CAD build for the part. Positions are in the model's coordinates, mm. Give positions to 0.01 mm unless a question says otherwise; leave off trailing zeros. Loops run counter-clockwise (first coordinate to the right, second up) from the corner with the lowest first, then second, coordinate; pieces in that order, holes last. Notation, with made-up numbers: M 88.5,-38.5 L 128.5,-38.5 A25 ccw 128.5,-18.5 Z; hole C -8.5,-9 d7. An arc over 180 degrees is marked long. Answer as CSV lines item,"result".
from build123d import *

# Parameters (mm, degrees)
F0_W         = 59.3232400715
F0_H         = 118.4509694576
F1_DEPTH     = 7.62
F2_T1_DEPTH  = 33.02
F3_T1_DEPTH  = 33.02
F4_T1_DEPTH  = 33.02
F5_T1_DEPTH  = 33.02
F17_W        = 8.8130328804
F17_H        = 2.5180093944
F18_DEPTH    = 0.254
F19_T1_DEPTH = 1.524
F20_R        = 0.508
F10_R        = 2.8607169915
F21_DEPTH    = 0.254
F11_R        = 2.8607134233
F22_DEPTH    = 0.254
F12_W        = 1.611137297
F12_H        = 7.3773153126
F23_DEPTH    = 0.254
F7_R         = 1.0781434008
F24_DEPTH    = 0.254
F9_W         = 6.8501718342
F9_H         = 1.6440376639
F25_DEPTH    = 0.254
F13_R        = 3.228368755
F26_DEPTH    = 0.254
F14_W        = 1.9021295011
F14_H        = 6.1539448798
F27_DEPTH    = 0.254
F8_R         = 3.0136808832
F28_DEPTH    = 0.254
F6_W         = 58.911472559
F6_H         = 101.9305512309
F29_DEPTH    = 0.254
F16_W        = 8.6615839973
F16_H        = 2.4723988026
F30_DEPTH    = 0.762
F15_R        = 2.8680658163
F31_DEPTH    = 0.762


# Not quite as in the source:
# - a fillet or chamfer that OpenCascade refuses, or shapes differently, is made with other operations: its cross-section is extruded or revolved along the edge and cut away or added


with BuildPart() as f1:
    # F0 (on Front) → F1 (new body)
    with BuildSketch(Plane.XZ):
        Rectangle(F0_W, F0_H)
    extrude(amount=F1_DEPTH)

    # F2: fillet of radius 5.08 on 1 edges, made by hand

    # F2_s2 → F2_t1 (cut)
    with BuildSketch(Plane.XZ.offset(-12.7)):
        with BuildLine():
            add(Edge.make_bspline(
                [(29.6616200358, 54.1454847288), (29.6616200358, 59.2254847288), (24.5816200358, 59.2254847288)],
                knots=[0, 0, 0, 1, 1, 1], degree=2, weights=[1, 1, 1]))
            Line((24.5816200358, 59.2254847288), (29.6616200358, 59.2254847288))
            Line((29.6616200358, 59.2254847288), (29.6616200358, 54.1454847288))
        make_face()
    extrude(amount=F2_T1_DEPTH, mode=Mode.SUBTRACT)

    # F3: fillet of radius 5.08 on 1 edges, made by hand

    # F3_s2 → F3_t1 (cut)
    with BuildSketch(Plane.XZ.offset(-12.7)):
        with BuildLine():
            add(Edge.make_bspline(
                [(-29.6616200358, 54.1454847288), (-29.6616200358, 59.2254847288), (-24.5816200358, 59.2254847288)],
                knots=[0, 0, 0, 1, 1, 1], degree=2, weights=[1, 1, 1]))
            Line((-24.5816200358, 59.2254847288), (-29.6616200358, 59.2254847288))
            Line((-29.6616200358, 59.2254847288), (-29.6616200358, 54.1454847288))
        make_face()
    extrude(amount=F3_T1_DEPTH, mode=Mode.SUBTRACT)

    # F4: fillet of radius 5.08 on 1 edges, made by hand

    # F4_s2 → F4_t1 (cut)
    with BuildSketch(Plane.XZ.offset(-12.7)):
        with BuildLine():
            add(Edge.make_bspline(
                [(-24.5816200358, -59.2254847288), (-29.6616200358, -59.2254847288), (-29.6616200358, -54.1454847288)],
                knots=[0, 0, 0, 1, 1, 1], degree=2, weights=[1, 1, 1]))
            Line((-29.6616200358, -54.1454847288), (-29.6616200358, -59.2254847288))
            Line((-29.6616200358, -59.2254847288), (-24.5816200358, -59.2254847288))
        make_face()
    extrude(amount=F4_T1_DEPTH, mode=Mode.SUBTRACT)

    # F5: fillet of radius 5.08 on 1 edges, made by hand

    # F5_s2 → F5_t1 (cut)
    with BuildSketch(Plane.XZ.offset(-12.7)):
        with BuildLine():
            add(Edge.make_bspline(
                [(29.6616200358, -54.1454847288), (29.6616200358, -59.2254847288), (24.5816200358, -59.2254847288)],
                knots=[0, 0, 0, 1, 1, 1], degree=2, weights=[1, 1, 1]))
            Line((24.5816200358, -59.2254847288), (29.6616200358, -59.2254847288))
            Line((29.6616200358, -59.2254847288), (29.6616200358, -54.1454847288))
        make_face()
    extrude(amount=F5_T1_DEPTH, mode=Mode.SUBTRACT)

    # F17 (on face) → F18 (join)
    with BuildSketch(Plane.XY.offset(59.2254847288)):
        with Locations((18.3535870165, -3.5715140402)):
            Rectangle(F17_W, F17_H)
    extrude(amount=F18_DEPTH)

    # F19: fillet of radius 0.508 on 1 edges, made by hand

    # F19_s2 → F19_t1 (cut)
    with BuildSketch(Plane.XY.offset(59.2254847288)):
        with BuildLine():
            add(Edge.make_bspline(
                [(22.2521034567, -2.312509343), (22.7601034567, -2.312509343), (22.7601034567, -2.820509343)],
                knots=[0, 0, 0, 1, 1, 1], degree=2, weights=[1, 1, 1]))
            Line((22.7601034567, -2.820509343), (22.7601034567, -2.312509343))
            Line((22.7601034567, -2.312509343), (22.2521034567, -2.312509343))
        make_face()
    extrude(amount=F19_T1_DEPTH, mode=Mode.SUBTRACT)

    # F20
    f20_edges = [f1.edges().sort_by_distance(p)[0] for p in [
        (13.947071, -2.312509, 59.352485),
        (22.760103, -4.830519, 59.352485),
        (13.947071, -4.830519, 59.352485),
    ]]
    fillet(f20_edges, radius=F20_R)

    # F10 (on face) → F21 (join)
    with BuildSketch(Plane(origin=(-29.6616200358, 0, 0), x_dir=(0, -1, 0), z_dir=(-1, 0, 0))):
        with Locations((3.9731003344, 38.3609607816)):
            Circle(F10_R)
    extrude(amount=F21_DEPTH)

    # F11 (on face) → F22 (join)
    with BuildSketch(Plane(origin=(-29.6616200358, 0, 0), x_dir=(0, -1, 0), z_dir=(-1, 0, 0))):
        with Locations((3.9731003344, 28.7707187235)):
            Circle(F11_R)
    extrude(amount=F22_DEPTH)

    # F12 (on face) → F23 (join)
    with BuildSketch(Plane(origin=(-29.6616200358, 0, 0), x_dir=(0, -1, 0), z_dir=(-1, 0, 0))):
        with Locations((3.8694504183, 49.0038786083)):
            Rectangle(F12_W, F12_H)
    extrude(amount=F23_DEPTH)

    # F7 (on face) → F24 (join)
    with BuildSketch(Plane(origin=(0, 0, 0), x_dir=(-1, 0, 0), z_dir=(0, 1, 0))):
        with Locations((0, 56.2707670033)):
            Circle(F7_R)
    extrude(amount=F24_DEPTH)

    # F9 (on face) → F25 (join)
    with BuildSketch(Plane(origin=(0, 0, 0), x_dir=(-1, 0, 0), z_dir=(0, 1, 0))):
        with Locations((0, 53.4313358366)):
            Rectangle(F9_W, F9_H)
    extrude(amount=F25_DEPTH)

    # F13 (on face) → F26 (join)
    with BuildSketch(Plane.XZ.offset(7.62)):
        with Locations((-22.3876349628, 54.8886656761)):
            Circle(F13_R)
    extrude(amount=F26_DEPTH)

    # F14 (on face) → F27 (join)
    with BuildSketch(Plane.XZ.offset(7.62)):
        with Locations((-16.1777436733, 55.0005566329)):
            Rectangle(F14_W, F14_H)
    extrude(amount=F27_DEPTH)

    # F8 (on Front) → F28 (join)
    with BuildSketch(Plane.XZ):
        with Locations((0, -55.3571693599)):
            Circle(F8_R)
    extrude(amount=-F28_DEPTH)

    # F6 (on Front) → F29 (join)
    with BuildSketch(Plane.XZ):
        Rectangle(F6_W, F6_H)
    extrude(amount=-F29_DEPTH)

    # F16 (on face) → F30 (cut)
    with BuildSketch(Plane(origin=(0, 0, -59.2254847288), x_dir=(1, 0, 0), z_dir=(0, 0, -1))):
        with Locations((0, 4.0924949571)):
            Rectangle(F16_W, F16_H)
    extrude(amount=-F30_DEPTH, mode=Mode.SUBTRACT)

    # F15 (on face) → F31 (cut)
    with BuildSketch(Plane(origin=(0, 0, -59.2254847288), x_dir=(1, 0, 0), z_dir=(0, 0, -1))):
        with Locations((19.5690467954, 3.8177834358)):
            Circle(F15_R)
    extrude(amount=-F31_DEPTH, mode=Mode.SUBTRACT)


solid = f1.part
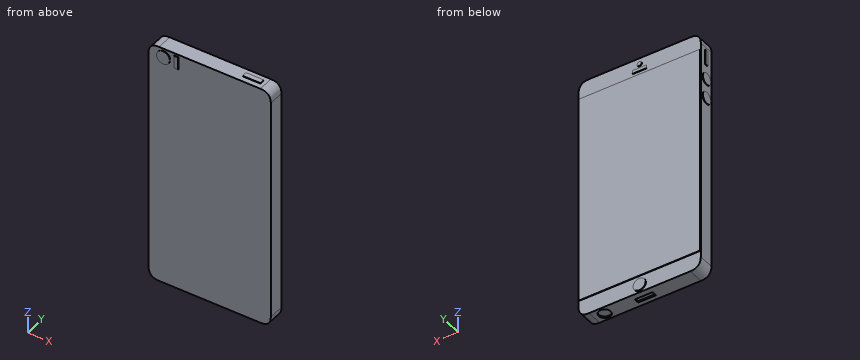
1) Drill centre lines: line 1 (Y direction, x = 21, z = -11.5); line 2 (X direction, y = -4.5, z = 53); line 3 (Z direction, x = 4, y = -0.25). Where is each one in solid material? Low to high. Write a range as from..to.
Answer below:
line 1,"y = -7.62..0.25"
line 2,"x = -29.66..29.66"
line 3,"z = -59.23..59.23"
2) Band-saw the part on B-B on z = -31.5. Give the cut face in (x, y).
Answer below:
outline,"M -29.66,-7.62 L 29.66,-7.62 L 29.66,0 L 29.46,0 L 29.46,0.25 L -29.46,0.25 L -29.46,0 L -29.66,0 Z"
3) Flat gauge pins, fed straight in: pin 1 (4 mm diameter, centred on x = -19.5, z = -9, fed in from -Y); pin 2 (1.7 mm diameter, centred on x = 18, y = -2.5, fed in from -Z). Where does each tip first touch, or does it go through?
Answer below:
pin 1,"stops at y = -7.62"
pin 2,"stops at z = -59.23"
4) Band-saw the part on A-A on x = 0. Give the cut face in (y, z).
Answer below:
outline,"M -7.62,-59.23 L -5.33,-59.23 L -5.33,-58.46 L -2.86,-58.46 L -2.86,-59.23 L 0,-59.23 L 0,-58.37 L 0.25,-58.37 L 0.25,-52.34 L 0,-52.34 L 0,-50.97 L 0.25,-50.97 L 0.25,50.97 L 0,50.97 L 0,52.61 L 0.25,52.61 L 0.25,54.25 L 0,54.25 L 0,55.19 L 0.25,55.19 L 0.25,57.35 L 0,57.35 L 0,59.23 L -7.62,59.23 Z"
